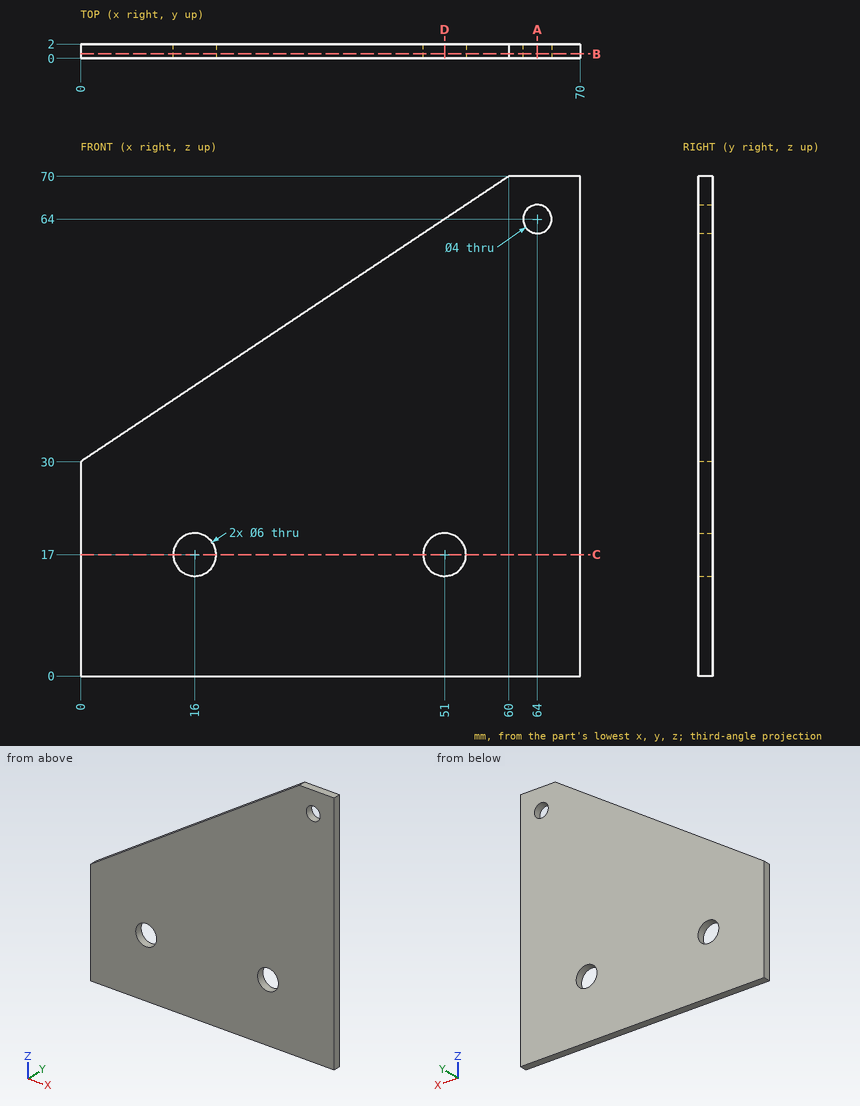
Answer from the drawing. Dimensions are ordinates in mm from the lowest x, y and z of the part. Give positions to 0.01 mm unless a question says otherwise; leave off trailing zeros. Write each loop counter-clockwise with the first axis right and the second up, starting at its lowest first coordinate (ties: lowest second). Pieces come first, ordered by that corner, then holes. Notation, with made-up numbers: (-31, -1.75) - (21, -1.75) arc R20 ccw to (21, 14.25) - close; hole circle Ø3 at (-26, -28). An arc over 180 degrees is marked (long way). One line per item, written item: value. Start each with the question number.
1. Consider probe 1 along Z at (x, y) = (64, 0.5); probe 2 along Z at (x, y) = (65, 0.6); probe 3 along X at (y, z) = (0.75, 60.5). Determine where each line is inside the solid, lowest interval first.
2. Find section A-A (x = 64). Write down the section's boundary in (y, z), then the cut area to 3 significant figures.
3. Find section C-C (z = 17). Write down the section's boundary in (x, y).
4. Find section B-B (y = 0.6). Write down the section's boundary in (x, z), then the cut area to 3 significant figures.
5. Find section D-D (x = 51). Write down the section's boundary in (y, z).
Geometry results:
1. probe 1: 0 to 62, 66 to 70
1. probe 2: 0 to 62.27, 65.73 to 70
1. probe 3: 45.75 to 70
2. outline: (0, 0) - (2, 0) - (2, 62) - (0, 62) - close; (0, 66) - (2, 66) - (2, 70) - (0, 70) - close
2. area: 132 mm2
3. outline: (0, 0) - (13, 0) - (13, 2) - (0, 2) - close; (19, 0) - (48, 0) - (48, 2) - (19, 2) - close; (54, 0) - (70, 0) - (70, 2) - (54, 2) - close
4. outline: (0, 0) - (70, 0) - (70, 70) - (60, 70) - (0, 30) - close; hole circle Ø6 at (16, 17); hole circle Ø6 at (51, 17); hole circle Ø4 at (64, 64)
4. area: 3,630 mm2
5. outline: (0, 0) - (2, 0) - (2, 14) - (0, 14) - close; (0, 20) - (2, 20) - (2, 64) - (0, 64) - close
